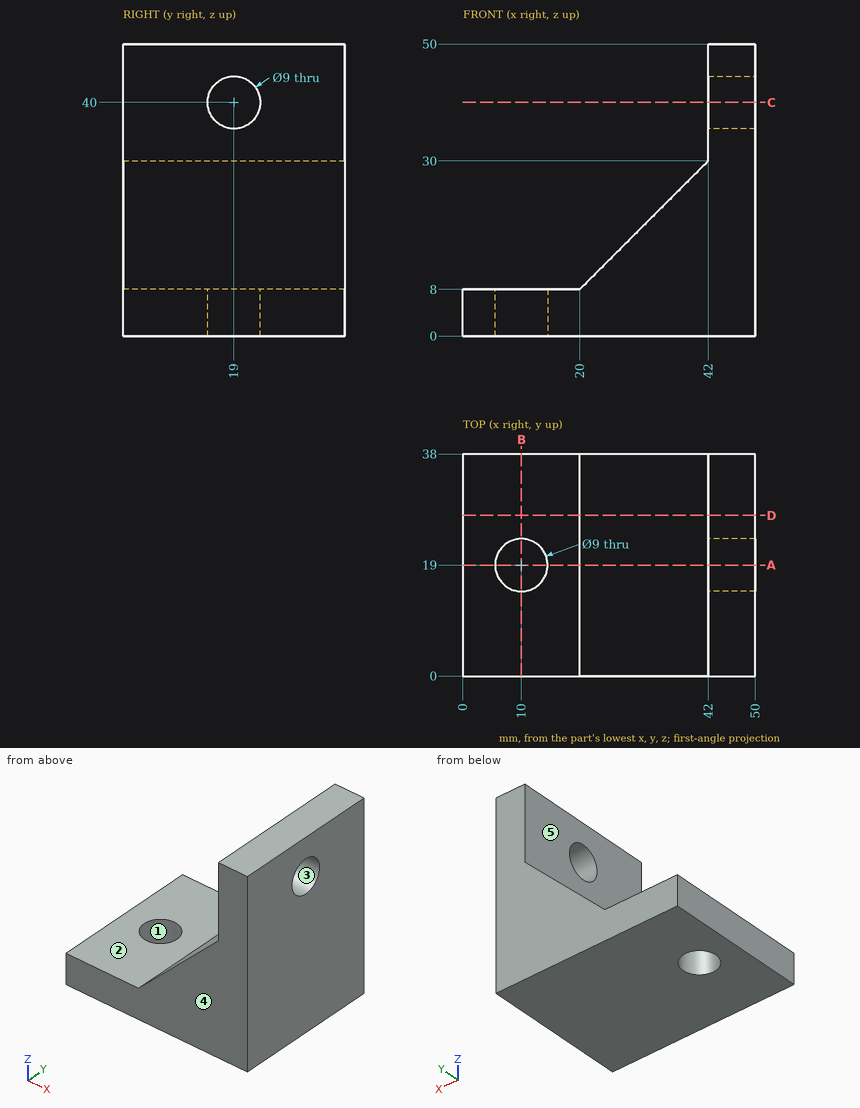
Check sheet for the drawn part. Datum: minimum x, y, z corner. Units: mm. A direction names the side the tool comes from. Coordinates: 2 decimals unless noted, no trailing zeros. Order: outer loops, then holes, each group sorted by start corner. A loop starts at its lowest first (then second) coordinate and runs counter-clockwise, first axis right, second up. Notation, with made-up numbers: M 27.5,59 L 61.5,59 A5 cw 61.5,63 Z; hole C -16.5,3.5 d1. An arc over 180 degrees is marked long. One line per question, with ' | ' between items. Start each with the question number.
Item 1: Cross-section at C-C on z = 40. Enter the section's corners in (x, y), then the cut area to 3 significant figures.
Item 2: Cross-section at A-A on y = 19. Enter the section's corners in (x, z).
Item 3: Draft check along Z on the marked faces 1, 2 and 3. Enter one of: pulls with the +Z half, pulls with the -Z half, needs draft (parallel to the pull), parting line crosses it, or undercut.
Item 4: Cross-section at D-D on y = 27.5. Enter the section's corners in (x, z), then the cut area to 3 significant figures.
Item 5: Set-up check for the marked faces 4 and 5: record each of +Z, -Z, +X, -X, +Y, -Y from which the full face is reachable in a straight line by a thin tool's end or side.
Item 6: Gauge pin test, flat ends, axial feed: pin 1 (22 mm diameter, centred on y = 23.5, z = 35.5, fed in from -X); pin 2 (14.5 mm diameter, centred on x = 10, y = 19, fed in from +Z); pin 3 (4 mm diameter, centred on y = 22.5, z = 42, fed in from -X). Record the tip position at first contact, or that the pin passes through.
Item 7: Material ranges on L1, parallel to Y at x = 44.75, z = 40; L2, parallel to Z at x = 12, y = 6; L3, parallel to X at y = 14, z = 42.5, recorded low to high. Write a range as [from, to].
Item 8: Cross-section at B-B on x = 10. Enter the section's corners in (y, z).
Findings:
1) outline: M 42,0 L 50,0 L 50,14.5 L 42,14.5 Z; M 42,23.5 L 50,23.5 L 50,38 L 42,38 Z | area: 232 mm²
2) outline: M 0,0 L 5.5,0 L 5.5,8 L 0,8 Z; M 14.5,0 L 50,0 L 50,35.5 L 42,35.5 L 42,30 L 20,8 L 14.5,8 Z; M 42,44.5 L 50,44.5 L 50,50 L 42,50 Z
3) face 1: needs draft | face 2: pulls with the +Z half | face 3: undercut
4) outline: M 0,0 L 50,0 L 50,50 L 42,50 L 42,30 L 20,8 L 0,8 Z | area: 978 mm²
5) face 4: +Z, -Z, +X, -X, -Y | face 5: +Z, -X, +Y, -Y
6) pin 1: stops at x = 36.5 | pin 2: stops at z = 8 | pin 3: stops at x = 42
7) L1: y = [0, 14.5], [23.5, 38] | L2: z = [0, 8] | L3: x = [42, 50]
8) outline: M 0,0 L 14.5,0 L 14.5,8 L 0,8 Z; M 23.5,0 L 38,0 L 38,8 L 23.5,8 Z
